Here's how the part is built. I have some questions about the finished solid (model axes, mm). A direction names the side the tool comes from. Give positions to 0.01 mm unless a question says otherwise; leave off trailing zeros. Loops run counter-clockwise (first coordinate to the right, second up) from the corner with the lowest first, then second, coordinate; pieces in that order, holes last.
Q1. We'd pull the mould along Y, two halves only. Please class faces 4 (the face through (0, 54, 0)), 5 (the face through (0.2, 24, 8.2)), 6 (the face through (-8, 46, 0)), 7 (the face through (5.46, 38, 6.06)): +Y half, -Y half, draft (parallel to the pull), parting line (faces both ways), or undercut.
Q2. If we section it at C-C (y = 27): Please give me the cut outline in (x, z), plus the area to 3 significant figures.
Q3. I need wall thicknesses on line 1 (X direction, y = 10.5, z = 0); line 2 (Y direction, x = -5.5, z = 7.5); line 3 (Y direction, x = -8.25, z = -4.5). Which ranges of each line are inside material? Lowest first, please.
Q4. If we section it at A-A (z = 1): Please give me the cut outline in (x, y), plus the area to 3 significant figures.
Q5. Will these pins go through, and if not, where does the flat tip stop? P1, Ø4, axis at x = 4, z = -4, coming from the -Y side; P2, Ø1.5, axis at y = 24.5, z = -6, coming from the +X side; P3, Ø8, axis at y = 49, z = 2, coming from the -X side; P4, Ø4, axis at y = 6.5, z = -2, coming from the +X side.
Q6. For faces 1 (the face through (0, 46, 8)), 2 (the face through (-1.73, 12.17, 7.81)), 3 (the face through (-1.73, 33.56, 7.81)), which set-ups out of +Z, -Z, +X, -X, +Y, -Y let a thin tool reach every point of the face, with its end or its side?
Q7. If we section it at B-B (y = 4): Please give me the cut outline in (x, z).
from build123d import *

# Parameters (mm, degrees)
SKETCH2_W           = 16
SKETCH2_H           = 16
BOSS_EXTRUDE1_DEPTH = 16


with BuildPart() as part:
    # Sketch1 → Revolve1 (revolve)
    with BuildSketch(Plane.XY):
        Polygon((0, 0), (8, 0), (8, 24), (12.5, 24), (12.5, 29), (8, 29), (8, 38), (0, 38), align=None)
    revolve(axis=Axis((0, 0, 0), (0, 1, 0)))

    # Sketch2 → Boss-Extrude1 (add)
    with BuildSketch(Plane(origin=(0, 38, 0), x_dir=(1, 0, 0), z_dir=(0, 1, 0))):
        Rectangle(SKETCH2_W, SKETCH2_H)
    extrude(amount=BOSS_EXTRUDE1_DEPTH)

    # Sketch3 → Cut-Revolve1 (revolve, cut)
    with BuildSketch(Plane(origin=(0, 0, 0), x_dir=(0.707106781, 0, -0.707106781), z_dir=(0.707106781, 0, 0.707106781))):
        with BuildLine():
            Line((11.313708499, 54), (8.313708499, 54))
            ThreePointArc((8.313708499, 54), (10.435028843, 53.121320344), (11.313708499, 51))
            Line((11.313708499, 51), (11.313708499, 54))
        make_face()
        with BuildLine():
            Line((11.313708499, 38), (8.313708499, 38))
            ThreePointArc((8.313708499, 38), (10.435028843, 38.878679656), (11.313708499, 41))
            Line((11.313708499, 41), (11.313708499, 38))
        make_face()
    revolve(axis=Axis((0, 34.971130997, 0), (0, -1, 0)), mode=Mode.SUBTRACT)


solid = part.part
Check sheet entries:
1. face 4: +Y half
1. face 5: -Y half
1. face 6: draft
1. face 7: undercut
2. outline: circle Ø25 at (0, 0)
2. area: 491 mm2
3. line 1: x = -8 to 8
3. line 2: y = 24 to 29, 38.17 to 53.83
3. line 3: y = 24 to 29
4. outline: (-12.46, 24) - (-7.94, 24) - (-7.94, 0) - (7.94, 0) - (7.94, 24) - (12.46, 24) - (12.46, 29) - (7.94, 29) - (7.94, 38) - (8, 38) - (8, 54) - (-8, 54) - (-8, 38) - (-7.94, 38) - (-7.94, 29) - (-12.46, 29) - close
4. area: 904 mm2
5. P1: stops at y = 0
5. P2: stops at x = 11.34
5. P3: stops at x = -8
5. P4: stops at x = 8
6. face 1: +Z, +X, -X, +Y
6. face 2: -Y
6. face 3: none
7. outline: circle Ø16 at (0, 0)
